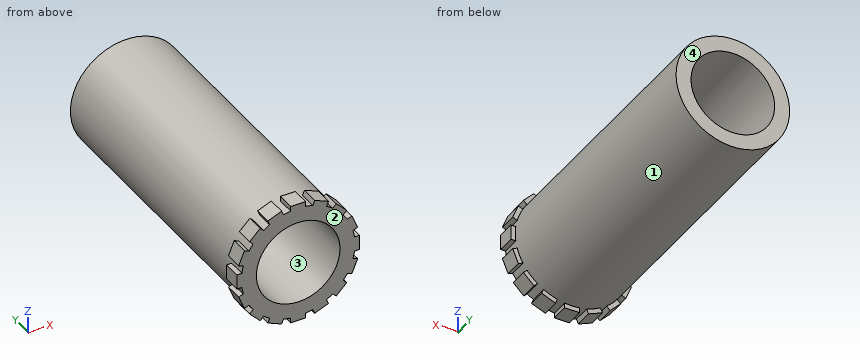
from build123d import *

# Parameters (mm, degrees)
SKETCH_1_R               = 9.5
SKETCH_1_R_2             = 7
EXTRUDE_1_DEPTH          = 50
SKETCH_2_W               = 1.5
SKETCH_2_H               = 2.5
EXTRUDE_2_DEPTH          = 3
PATTERN_CIRCULAR_1_COUNT = 16


with BuildPart() as part:
    # 草图1 → 凸台-拉伸1 (new body)
    with BuildSketch(Plane(origin=(0, 0, 0), x_dir=(1, 0, 0), z_dir=(0, 1, 0))):
        Circle(SKETCH_1_R)
        Circle(SKETCH_1_R_2, mode=Mode.SUBTRACT)
    extrude(amount=EXTRUDE_1_DEPTH)

    # 草图2 → 凸台-拉伸2 (add)
    with BuildSketch(Plane(origin=(0, 0, 0), x_dir=(-1, 0, 0), z_dir=(0, -1, 0))):
        with Locations((9.5, 0)):
            Rectangle(SKETCH_2_W, SKETCH_2_H)
    extrude_2 = extrude(amount=-EXTRUDE_2_DEPTH)

    # 阵列(圆周)1: 凸台-拉伸2 ×16 about axis
    pattern_circular_1_axis = Axis((0, 0, 0), (0, 1, 0))
    for i in range(1, PATTERN_CIRCULAR_1_COUNT):
        add(extrude_2.rotate(pattern_circular_1_axis, i * 360 / PATTERN_CIRCULAR_1_COUNT))


solid = part.part
Geometry: final body of the model. Coordinates: model frame, mm. Face numbers are marked on the shaded views. A direction names the side the tool comes from. Give positions to 0.01 mm unless a question says otherwise; leave off trailing zeros. Order: outer loops, then holes, each group sorted by start corner. A loop starts at its lowest first (then second) coordinate and runs counter-clockwise, first axis right, second up. Notation, with made-up numbers: (-13.75, 33.5) - (15.25, 33.5) arc R20 cw to (15.25, 39.5) - close; hole circle Ø5 at (56.25, 48.5). An arc over 180 degrees is marked (long way). Use CSV: the item, a comma, the result in double quotes.
1. Material intervals for line 1 along X through (y, z) = (23, 0); line 2 along Z through (x, y) = (2.5, 18), sorted ascending. Write a range as from..to.
Answers below:
line 1,"-9.5..-7, 7..9.5"
line 2,"-9.17..-6.54, 6.54..9.17"
2. Mould query, pull axis X, two halves, no side actions, for the marked faces 3 and 4. Classes: +X half, -X half, draft (parallel to the pull), parting line (faces both ways), or undercut.
Answers below:
face 3,"undercut"
face 4,"draft"
3. Section query B-B (z = 0). Output: boundary loops of the cut face in (x, y), plus the area to 4 significant figures.
Answers below:
outline,"(-10.25, 0) - (-7, 0) - (-7, 50) - (-9.5, 50) - (-9.5, 3) - (-10.25, 3) - close; (7, 0) - (10.25, 0) - (10.25, 3) - (9.5, 3) - (9.5, 50) - (7, 50) - close"
area,"254.5 mm2"
4. Contact query for flat-ended pins moving along their axis: pin 1 (12 mm diameter, centred on y = 18.5, z = 4.5, fed in from +X); pin 2 (6 mm diameter, centred on x = 7.5, y = 37.5, fed in from -Z); pin 3 (10 mm diameter, centred on x = 5, y = 14, fed in from +Z). Output: stop coordinate, or through.
Answers below:
pin 1,"x = 9.5"
pin 2,"z = -8.37"
pin 3,"z = 9.5"
5. Section query C-C (y = 11). Output: boundary loops of the cut face in (x, z).
Answers below:
outline,"circle Ø19 at (0, 0); hole circle Ø14 at (0, 0)"
6. Access query for the marked faces 1 and 2. Directions: +Z, -Z, +X, -X, +Y, -Y. A direction counts if a zero-diameter tool reaches every point of the face in a straight line with its end or side. Return the directions, or none.
Answers below:
face 1,"+Y"
face 2,"+Z, -Z, +X, -X, -Y"
7. Section query A-A (x = 0). Output: boundary loops of the cut face in (y, z), plus the area to 4 significant figures.
Answers below:
outline,"(0, -10.25) - (3, -10.25) - (3, -9.5) - (50, -9.5) - (50, -7) - (0, -7) - close; (0, 7) - (50, 7) - (50, 9.5) - (3, 9.5) - (3, 10.25) - (0, 10.25) - close"
area,"254.5 mm2"
